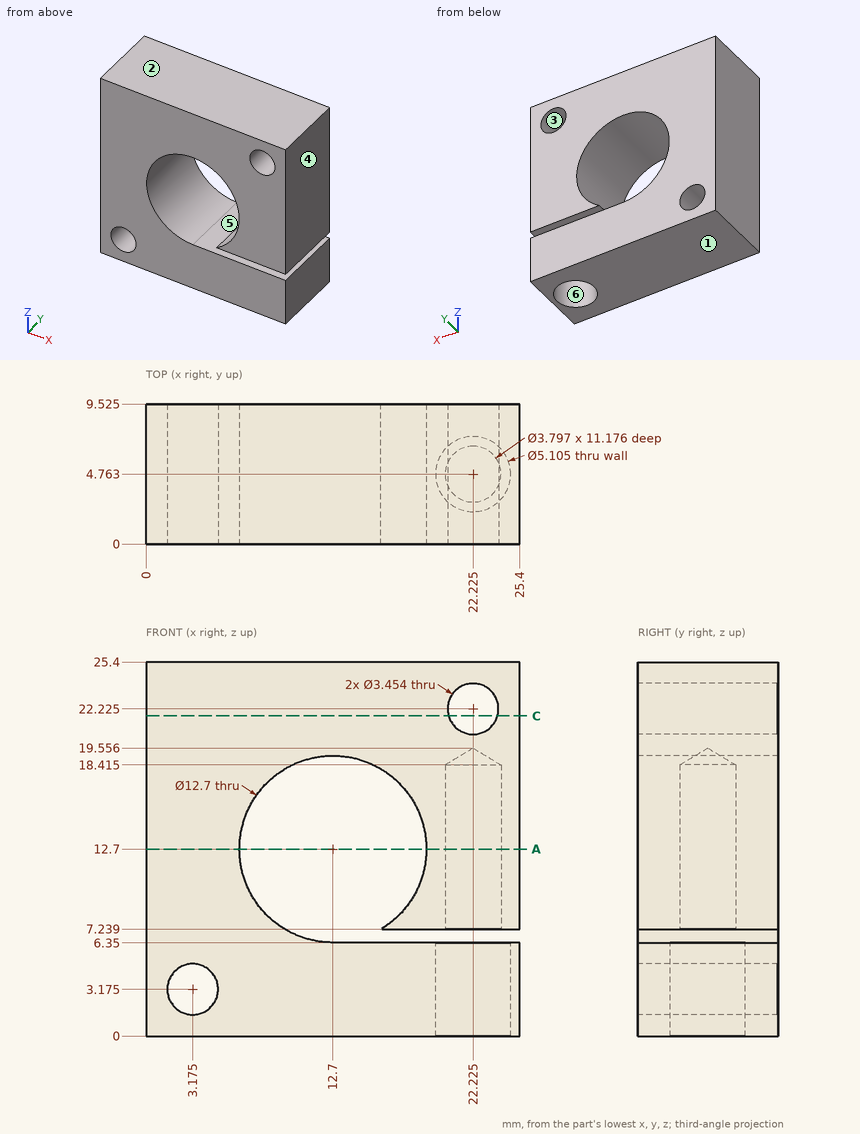
Check sheet for the drawn part. Datum: minimum x, y, z corner. Units: mm. A direction names the side the tool comes from. Round coordinates to 2 decimals unless told otherwise and drop trailing zeros. Order: outer loops, then holes, each group sorted by start corner. A loop starts at its lowest first (then second) coordinate and runs counter-clockwise, first axis right, second up. Notation, with made-up numbers: (48.5, -5) -> (98.5, -5) arc R34 ccw to (98.5, 32) -> close; hole circle Ø1 at (29, 76). An arc over 180 degrees is marked (long way). Return JSON: item names as keys, results as strings. Group by question number.
Q1. Material ranges on probe 1 along Z at (x, y) = (17.25, 2); probe 2 along Z at (x, y) = (8.75, 2); probe 3 along X at (y, z) = (5, 2.75), recorded low to high. Write a range as from..to.
Q2. Tool access check on the marked faces 4, 5 and 6. Record the directions out of +Z, -Z, +X, -X, +Y, -Y that give a thin tool (end or side, any length) a straight path to the whole face; none if there is none.
Q3. Section check C-C, the plane z = 21.75. Record the boundary of the cut face in (x, y) (1 decimal), plus the area to 3 significant figures.
Q4. Gauge pin test, flat ends, axial feed: pin 1 (1.5 mm diameter, centred on x = 17, y = 7, fed in from -Z); pin 2 (3 mm diameter, centred on x = 22.5, y = 5.5, fed in from -Z). Record the tip position at first contact, or that the pin passes through.
Q5. Section check A-A, the plane z = 12.7. Count the separate pieces of the cut face and the enclosed holes in it, plus the area to 3 significant figures.
Q6. Release check for a two-part mould opening along Z. For the marked faces 1, 2 and 3 record: released by +Z, released by -Z, zero draft, split by the parting line, or undercut.
Numbers:
{
 "1": {"probe 1": "0..6.35, 7.24..8.27, 17.13..25.4", "probe 2": "0..7.73, 17.67..25.4", "probe 3": "0..1.5, 4.85..19.68, 24.77..25.4"},
 "2": {"face 4": "+Z, -Z, +X, +Y, -Y", "face 5": "+X, +Y, -Y", "face 6": "-Z"},
 "3": {"outline": "(0, 0) -> (20.6, 0) -> (20.6, 9.5) -> (0, 9.5) -> close; (23.9, 0) -> (25.4, 0) -> (25.4, 9.5) -> (23.9, 9.5) -> close", "area": "210 mm^2"},
 "4": {"pin 1": "z = 0", "pin 2": "z = 7.24"},
 "5": {"separate pieces": "2", "enclosed holes": "1", "area": "110 mm^2"},
 "6": {"face 1": "released by -Z", "face 2": "released by +Z", "face 3": "undercut"}
}
